from build123d import *

# Parameters (mm, degrees)
SKETCH1_W               = 255
SKETCH1_H               = 150
BOSS_EXTRUDE1_DEPTH     = 3
SKETCH3_R               = 29
CUT_EXTRUDE2_DEPTH      = 3
CUT_EXTRUDE3_REACH      = 149.954
SKETCH4_R               = 1.6
SKETCH5_W               = 15
SKETCH5_H               = 6
BOSS_EXTRUDE2_DEPTH     = 9.8
CUT_EXTRUDE4_REACH      = 184.352
SKETCH6_R               = 4
SKETCH7_R               = 5
CUT_EXTRUDE5_DEPTH      = 2
SKETCH8_W               = 15
SKETCH8_H               = 18
SKETCH8_H_2             = 6
BOSS_EXTRUDE3_DEPTH     = 9.8
SKETCH9_R               = 4
CUT_EXTRUDE6_DEPTH      = 24
SKETCH10_R              = 5
CUT_EXTRUDE7_DEPTH      = 2
LPATTERN1_COUNT         = 2
LPATTERN1_PITCH         = 18
MIRROR2_COPY_1_SKETCH_R = 5
MIRROR2_COPY_1_DEPTH    = 2
CHAMFER1_SIZE           = 2
F_4_0MM_DOWEL_HOLE1_D   = 4


with BuildPart() as part:
    # Sketch1 → Boss-Extrude1 (new body)
    with BuildSketch(Plane(origin=(0, 0, 0), x_dir=(1, 0, 0), z_dir=(0, 1, 0))):
        Rectangle(SKETCH1_W, SKETCH1_H)
    extrude(amount=BOSS_EXTRUDE1_DEPTH)

    # Sketch3 → Cut-Extrude2 (cut)
    with BuildSketch(Plane(origin=(0, 3, 0), x_dir=(1, 0, 0), z_dir=(0, 1, 0))):
        with Locations(Location((17.5, 0, 0), (0, 0, 270))):
            Circle(SKETCH3_R)
    extrude(amount=-CUT_EXTRUDE2_DEPTH, mode=Mode.SUBTRACT)

    # Sketch4 → Cut-Extrude3 (cut, up to next)
    with BuildSketch(Plane(origin=(0, 3, 0), x_dir=(1, 0, 0), z_dir=(0, 1, 0)), mode=Mode.PRIVATE) as cut_extrude3_sk1:
        with Locations(Location((-72.421312687, -3.64086936, 0), (0, 0, 270))):
            Circle(SKETCH4_R)
    cut_extrude3_tool1 = extrude(cut_extrude3_sk1.sketch, amount=-CUT_EXTRUDE3_REACH, mode=Mode.PRIVATE) & part.part
    # Sketch4 → Cut-Extrude3 (cut, up to next)
    with BuildSketch(Plane(origin=(0, 3, 0), x_dir=(1, 0, 0), z_dir=(0, 1, 0)), mode=Mode.PRIVATE) as cut_extrude3_sk2:
        with Locations(Location((-72.421312687, 26.99913064, 0), (0, 0, 270))):
            Circle(SKETCH4_R)
    cut_extrude3_tool2 = extrude(cut_extrude3_sk2.sketch, amount=-CUT_EXTRUDE3_REACH, mode=Mode.PRIVATE) & part.part
    # Sketch4 → Cut-Extrude3 (cut, up to next)
    with BuildSketch(Plane(origin=(0, 3, 0), x_dir=(1, 0, 0), z_dir=(0, 1, 0)), mode=Mode.PRIVATE) as cut_extrude3_sk3:
        with Locations(Location((-114.421312687, -3.64086936, 0), (0, 0, 270))):
            Circle(SKETCH4_R)
    cut_extrude3_tool3 = extrude(cut_extrude3_sk3.sketch, amount=-CUT_EXTRUDE3_REACH, mode=Mode.PRIVATE) & part.part
    # Sketch4 → Cut-Extrude3 (cut, up to next)
    with BuildSketch(Plane(origin=(0, 3, 0), x_dir=(1, 0, 0), z_dir=(0, 1, 0)), mode=Mode.PRIVATE) as cut_extrude3_sk4:
        with Locations(Location((-114.421312687, 26.99913064, 0), (0, 0, 270))):
            Circle(SKETCH4_R)
    cut_extrude3_tool4 = extrude(cut_extrude3_sk4.sketch, amount=-CUT_EXTRUDE3_REACH, mode=Mode.PRIVATE) & part.part
    add(cut_extrude3_tool1.solids().sort_by_distance((-72.421313, 3, 3.640869))[0], mode=Mode.SUBTRACT)
    add(cut_extrude3_tool2.solids().sort_by_distance((-72.421313, 3, -26.999131))[0], mode=Mode.SUBTRACT)
    add(cut_extrude3_tool3.solids().sort_by_distance((-114.421313, 3, 3.640869))[0], mode=Mode.SUBTRACT)
    add(cut_extrude3_tool4.solids().sort_by_distance((-114.421313, 3, -26.999131))[0], mode=Mode.SUBTRACT)

    # Sketch5 → Boss-Extrude2 (add)
    with BuildSketch(Plane(origin=(0, 0, 0), x_dir=(1, 0, 0), z_dir=(0, 1, 0))):
        with Locations((-114.9, -52)):
            Rectangle(SKETCH5_W, SKETCH5_H)
    boss_extrude2 = extrude(amount=-BOSS_EXTRUDE2_DEPTH)

    # Sketch6 → Cut-Extrude4 (cut, up to next)
    with BuildSketch(Plane.XY.offset(55), mode=Mode.PRIVATE) as cut_extrude4_sk1:
        with Locations((-114.9, -9.8)):
            Circle(SKETCH6_R)
    cut_extrude4_tool1 = extrude(cut_extrude4_sk1.sketch, amount=-CUT_EXTRUDE4_REACH, mode=Mode.PRIVATE) & part.part
    cut_extrude4 = cut_extrude4_tool1.solids().sort_by_distance((-114.9, -9.8, 55))[0]
    add(cut_extrude4, mode=Mode.SUBTRACT)

    # Sketch7 → Cut-Extrude5 (cut, symmetric)
    with BuildSketch(Plane.XY.offset(52)):
        with Locations((-114.9, -9.8)):
            Circle(SKETCH7_R)
    cut_extrude5 = extrude(amount=CUT_EXTRUDE5_DEPTH, both=True, mode=Mode.SUBTRACT)

    # Mirror1: Boss-Extrude2, Cut-Extrude4, Cut-Extrude5 across plane
    add(boss_extrude2.mirror(Plane.XY))
    add(cut_extrude4.mirror(Plane.XY), mode=Mode.SUBTRACT)
    add(cut_extrude5.mirror(Plane.XY), mode=Mode.SUBTRACT)

    # Sketch8 → Boss-Extrude3 (add)
    with BuildSketch(Plane.XZ):
        with Locations((120, -61)):
            Rectangle(SKETCH8_W, SKETCH8_H)
        with Locations((120, -37)):
            Rectangle(SKETCH8_W, SKETCH8_H_2)
    boss_extrude3 = extrude(amount=BOSS_EXTRUDE3_DEPTH)

    # Sketch9 → Cut-Extrude6 (cut)
    with BuildSketch(Plane.XY.offset(-34)):
        with Locations((120, -9.8)):
            Circle(SKETCH9_R)
    cut_extrude6 = extrude(amount=-CUT_EXTRUDE6_DEPTH, mode=Mode.SUBTRACT)

    # Sketch10 → Cut-Extrude7 (cut, symmetric)
    with BuildSketch(Plane.XY.offset(-37)):
        with Locations((120, -9.8)):
            Circle(SKETCH10_R)
    cut_extrude7 = extrude(amount=CUT_EXTRUDE7_DEPTH, both=True, mode=Mode.SUBTRACT)

    # LPattern1: Cut-Extrude7 ×2
    with Locations(*[(0, 0, -i * LPATTERN1_PITCH) for i in range(1, LPATTERN1_COUNT)]):
        add(cut_extrude7, mode=Mode.SUBTRACT)

    # Mirror2: Boss-Extrude3, Cut-Extrude6, Cut-Extrude7 across plane
    add(boss_extrude3.mirror(Plane.XY))
    add(cut_extrude6.mirror(Plane.XY), mode=Mode.SUBTRACT)
    add(cut_extrude7.mirror(Plane.XY), mode=Mode.SUBTRACT)

    # Mirror2 copy 1 sketch → Mirror2 copy 1 (cut, symmetric)
    with BuildSketch(Plane(origin=(0, 0, 55), x_dir=(1, 0, 0), z_dir=(0, 0, -1))):
        with Locations((120, 9.8)):
            Circle(MIRROR2_COPY_1_SKETCH_R)
    extrude(amount=MIRROR2_COPY_1_DEPTH, both=True, mode=Mode.SUBTRACT)

    # Chamfer1
    chamfer1_edges = [part.edges().sort_by_distance(p)[0] for p in [
        (17.5, 0, -29),
    ]]
    chamfer(chamfer1_edges, length=CHAMFER1_SIZE)

    # Ø4.0mm Dowel Hole1 (through all)
    with Locations(Plane(origin=(0, 3, 0), x_dir=(1, 0, 0), z_dir=(0, 1, 0))):
        with Locations((119.5, -63), (119.5, 63)):
            f_4_0mm_dowel_hole1 = Hole(F_4_0MM_DOWEL_HOLE1_D / 2)

    # Mirror3: Ø4.0mm Dowel Hole1 across plane
    add(f_4_0mm_dowel_hole1.mirror(Plane(origin=(0, 0, 0), x_dir=(0, 0, 1), z_dir=(1, 0, 0))), mode=Mode.SUBTRACT)


solid = part.part
Read the model definition and answer for the solid it produces. Units are mm, in the model's axes. A direction names the side the tool comes from. Coordinates: 2 decimals unless noted, no trailing zeros. Write each loop counter-clockwise with the first axis right and the second up, starting at its lowest first coordinate (ties: lowest second). Pieces come first, ordered by that corner, then holes. Notation, with made-up numbers: (55, 17) -> (61, 17) arc R23 ccw to (61, 51) -> close; hole circle Ø2 at (29, 43). An arc over 180 degrees is marked (long way). Return JSON: item names as keys, results as strings.
(1) The part is cut by section D-D on x = -68. Give the vertices of the cut face in (y, z).
Answers below:
{"outline": "(0, -75) -> (3, -75) -> (3, 75) -> (0, 75) -> close"}
(2) Which of the six approach directions +Z, -Z, +X, -X, +Y, -Y give full straight-line access (tool end or side, diameter ignored) to faces 4 (the flat face through (-115, -4, 49)), 5 (the cylindrical face through (120.1, -4.8, -55)), 6 (the flat face through (112.5, -5, 37)), 7 (the flat face through (120, -4, -52)), 8 (the flat face through (119.9, -9.8, 60.87))?
Answers below:
{"face 4": "+X, -X, -Y", "face 5": "-Y", "face 6": "+Z, -Z, -X, -Y", "face 7": "+X, -Y", "face 8": "+Z, -Z, +X, -X, -Y"}
(3) The part is cut by section A-A on y = -2.5. Give the vertices of the cut face in (x, z), then the cut area to 3 significant figures.
Answers below:
{"outline": "(-122.4, -55) -> (-107.4, -55) -> (-107.4, -49) -> (-122.4, -49) -> close; (-122.4, 49) -> (-107.4, 49) -> (-107.4, 55) -> (-122.4, 55) -> close; (112.5, -70) -> (127.5, -70) -> (127.5, -52) -> (112.5, -52) -> close; (112.5, -40) -> (127.5, -40) -> (127.5, -34) -> (112.5, -34) -> close; (112.5, 34) -> (127.5, 34) -> (127.5, 40) -> (112.5, 40) -> close; (112.5, 52) -> (127.5, 52) -> (127.5, 70) -> (112.5, 70) -> close; hole circle Ø4 at (119.5, -63); hole circle Ø4 at (119.5, 63)", "area": "875 mm^2"}
(4) The part is cut by section C-C on z = 45.5. Give the vertices of the cut face in (x, y).
Answers below:
{"outline": "(-127.5, 0) -> (127.5, 0) -> (127.5, 3) -> (-127.5, 3) -> close"}
(5) Consider line 1 along Z through (x, y) = (119.5, -4.5); line 2 along X through (y, z) = (-0.5, 53); line 3 along Y through (x, z) = (58.5, -43.5). Determine where each line is inside the solid, lowest interval first. Write a range as from..to.
Answers below:
{"line 1": "-70..-65, -61..-52, -40..-34, 34..40, 52..61, 65..70", "line 2": "-122.4..-107.4, 112.5..127.5", "line 3": "0..3"}
(6) Each of these flat-tipped pins is pushed along its axis until it touches: P1, Ø5.5, axis at x = 119.5, y = -7.5, coming from the -Z side; P2, Ø6.5, axis at x = -119.5, z = 63, coming from the +Y side; P3, Ø2.5, axis at x = 120.5, y = -8, coming from the +Z side; P4, Ø3, axis at x = -119.5, z = -63, coming from the -Y side. Where does it stop, or does it pass through?
Answers below:
{"P1": "z = -70", "P2": "y = 3", "P3": "z = 70", "P4": "through"}
(7) The part is cut by section B-B on x = 17.5. Give the vertices of the cut face in (y, z).
Answers below:
{"outline": "(0, -75) -> (3, -75) -> (3, -29) -> (2, -29) -> (0, -31) -> close; (0, 31) -> (2, 29) -> (3, 29) -> (3, 75) -> (0, 75) -> close"}
(8) For a pull along Z with two mould halves and no side action, classify faces 1 (the flat face through (120, -4, 52)), 2 (the flat face through (112.5, -5, -61)), 3 (the flat face through (120, -5, -70)) as pulls with the +Z half, pulls with the -Z half, needs draft (parallel to the pull), parting line crosses it, or undercut.
Answers below:
{"face 1": "undercut", "face 2": "needs draft", "face 3": "pulls with the -Z half"}
